Build history of the part. All positions in model axes, mm. A direction names the side the tool comes from. Round coordinates to 2 decimals unless told otherwise and drop trailing zeros. Write each loop counter-clockwise with the first axis right and the second up, starting at its lowest first coordinate (ties: lowest second). Pieces come first, ordered by that corner, then holes. Notation, with made-up numbers: (-13, 50) -> (11, 50) arc R25 ccw to (11, 78) -> close; hole circle Ø8 at (60, 86.5). An arc over 180 degrees is marked (long way). One line per question, with ' | ' between items.
from build123d import *

# Parameters (mm, degrees)
SKIZZE1_W                       = 15
SKIZZE1_H                       = 19
AUFSATZ_LINEAR_AUSTRAGEN1_DEPTH = 3
AUFSATZ_LINEAR_AUSTRAGEN2_DEPTH = 19
SKIZZE5_R                       = 3
SCHNITT_LINEAR_AUSTRAGEN1_DEPTH = 3
SKIZZE6_W                       = 15
SKIZZE6_H                       = 19
AUFSATZ_LINEAR_AUSTRAGEN3_DEPTH = 0.5
SKIZZE7_W                       = 15.231399179
SKIZZE7_H                       = 1.8
AUFSATZ_LINEAR_AUSTRAGEN4_DEPTH = 3.6
AUFSATZ_LINEAR_AUSTRAGEN5_DEPTH = 1.8
AUFSATZ_LINEAR_AUSTRAGEN6_DEPTH = 1.8


with BuildPart() as part:
    # Skizze1 → Aufsatz-Linear austragen1 (new body)
    with BuildSketch(Plane.XY):
        Rectangle(SKIZZE1_W, SKIZZE1_H)
    extrude(amount=AUFSATZ_LINEAR_AUSTRAGEN1_DEPTH)

    # Skizze3 → Aufsatz-Linear austragen2 (add)
    with BuildSketch(Plane(origin=(0, 9.5, 0), x_dir=(1, 0, 0), z_dir=(0, 1, 0))):
        Polygon((-7.5, 0), (-7.5, 2.644904711), (7.5, 0), align=None)
    extrude(amount=-AUFSATZ_LINEAR_AUSTRAGEN2_DEPTH)

    # Skizze5 → Schnitt-Linear austragen1 (cut)
    with BuildSketch(Plane.XY.offset(3)):
        Circle(SKIZZE5_R)
    extrude(amount=-SCHNITT_LINEAR_AUSTRAGEN1_DEPTH, mode=Mode.SUBTRACT)

    # Skizze6 → Aufsatz-Linear austragen3 (add)
    with BuildSketch(Plane.XY.offset(3)):
        Rectangle(SKIZZE6_W, SKIZZE6_H)
    extrude(amount=AUFSATZ_LINEAR_AUSTRAGEN3_DEPTH)

    # Skizze7 → Aufsatz-Linear austragen4 (add)
    with BuildSketch(Plane(origin=(0.226152672, 0, -1.282575537), x_dir=(-0.984807753, 0, -0.173648178), z_dir=(0.173648178, 0, -0.984807753))):
        with Locations((0.229641442, 8.6)):
            Rectangle(SKIZZE7_W, SKIZZE7_H)
        with Locations((0.229641442, -8.6)):
            Rectangle(SKIZZE7_W, SKIZZE7_H)
    extrude(amount=AUFSATZ_LINEAR_AUSTRAGEN4_DEPTH)

    # Skizze10 → Aufsatz-Linear austragen5 (add)
    with BuildSketch(Plane.XZ.offset(-7.7)):
        Polygon((8.12513344, -3.545307911), (7.81256672, -1.772653955), (-7.18743328, -4.417558666), (-6.87486656, -6.190212621), align=None)
    extrude(amount=AUFSATZ_LINEAR_AUSTRAGEN5_DEPTH)

    # Skizze9 → Aufsatz-Linear austragen6 (add)
    with BuildSketch(Plane(origin=(0, -7.7, 0), x_dir=(1, 0, 0), z_dir=(0, 1, 0))):
        Polygon((7.81256672, 1.772653955), (-7.18743328, 4.417558666), (-6.87486656, 6.190212621), (8.12513344, 3.545307911), align=None)
    extrude(amount=AUFSATZ_LINEAR_AUSTRAGEN6_DEPTH)


solid = part.part
(1) Drop flat-ended pins along their axis: pin 1 (2 mm diameter, centred on y = 0, z = 2, fed in from +X); pin 2 (5 mm diameter, centred on x = -1, y = -0.5, fed in from -Z); pin 3 (1.5 mm diameter, centred on x = -1, y = -2.5, fed in from -Z). Give the stop position or say it passes through.
Calculated:
pin 1: x = 7.5 | pin 2: z = -1.94 | pin 3: z = -1.63
(2) Slice it at C-C (x = 1). Write the cut outline in (y, z), then the cut area to 3 significant figures.
Calculated:
outline: (-9.5, -4.8) -> (-5.9, -4.8) -> (-5.9, -2.97) -> (-7.7, -2.97) -> (-7.7, -1.15) -> (7.7, -1.15) -> (7.7, -2.97) -> (5.9, -2.97) -> (5.9, -4.8) -> (9.5, -4.8) -> (9.5, 3.5) -> (-9.5, 3.5) -> close; hole (-2.83, 0) -> (2.83, 0) -> (2.83, 3) -> (-2.83, 3) -> close | area: 91.0 mm2
(3) Wall check: line 1 (Y direction, x = 0, z = 1); line 2 (Y direction, x = -1, z = -3.75); line 3 (X direction, y = 8.5, z = 0.5). Give the ranges that are in metal, low to high. Write a range as from..to.
Calculated:
line 1: -9.5..-3, 3..9.5 | line 2: -9.5..-5.9, 5.9..9.5 | line 3: -7.5..7.5
(4) Mould opens along Z. For faces 5 (the flat face through (0, 0, 3.5)), 6 (the flat face through (-0.11, 0.11, -1.34)), 7 (the flat face through (0, 9.5, -1)) say: pulls with the +Z half, pulls with the -Z half, needs draft (parallel to the pull), parting line crosses it, or undercut.
Calculated:
face 5: pulls with the +Z half | face 6: undercut | face 7: needs draft
(5) 3-axis set-ups, long thin cutter, end or side, ignore diameter. For faces 1 (the flat face through (-7.5, 0, 0)), 2 (the flat face through (0, -9.5, 0)), 3 (the flat face through (7.5, 0, 2)), 4 (the cylindrical face through (-3, 0, 2)): which of +Z, -Z, +X, -X, +Y, -Y reach the whole face in a straight line?
Calculated:
face 1: +Z, -Z, -X, +Y, -Y | face 2: +Z, -Z, +X, -X, -Y | face 3: +Z, +X, +Y, -Y | face 4: none
(6) Slice it at B-B (z = 1.75). Write the cut outline in (x, y), then the cut area to 3 significant figures.
Calculated:
outline: (-7.5, -9.5) -> (7.5, -9.5) -> (7.5, 9.5) -> (-7.5, 9.5) -> close; hole circle Ø6 at (0, 0) | area: 257 mm2
(7) Slice it at D-D (y = -5.5). Write the cut outline in (x, z).
Calculated:
outline: (-7.5, -2.64) -> (7.5, 0) -> (7.5, 3.5) -> (-7.5, 3.5) -> close
(8) Slice it at A-A (y = 0). Write the cut outline in (x, z).
Calculated:
outline: (-7.5, -2.64) -> (7.5, 0) -> (7.5, 3.5) -> (-7.5, 3.5) -> close; hole (-3, 0) -> (3, 0) -> (3, 3) -> (-3, 3) -> close
